Autodesk Inventor part; units mm, degrees
ref_plane "Work Plane2" through (0, 10, 0) normal (0, 1, 0) x (1, 0, 0)
ref_plane "YZ Plane" through (0, 0, 0) normal (1, 0, 0) x (0, 1, 0)
ref_plane "XZ Plane" through (0, 0, 0) normal (0, 1, 0) x (-1, 0, 0)
sketch "Sketch1" plane through (0, 0, 0) normal (0, 1, 0) x (-1, 0, 0)
  circle A0 centre (0, 0) radius 66
  circle A1 centre (0, 0) radius 61
  circle A2 centre (0, 0) radius 59
  dimension "Absolute_Diameter" = 132
  dimension "Diameter_No_Outer_Lip" = 122
  dimension "Inner_Cylinder_Diameter" = 118
extrude "Extrusion1" add sketch "Sketch1" along normal blind 4 contours A0
extrude "Extrusion2" add sketch "Sketch1" along normal blind 75 contours A1
sketch "Sketch2" plane through (0, 75, 0) normal (0, 1, 0) x (1, 0, 0)
  circle A0 centre (0, 0) radius 40.5
  circle A1 centre (0, 0) radius 61
  dimension "Lip_Diameter_Out" = 81
  dimension "Top_Outer_Lip_Diameter" = 122
extrude "Extrusion7" add sketch "Sketch2" against normal blind 8
ref_plane "Work Plane2" through (0, 10, 0) normal (0, 1, 0) x (1, 0, 0)
sketch "Sketch3" plane through (0, 10, 0) normal (0, 1, 0) x (1, 0, 0)
  circle A0 centre (0, 0) radius 127.5
  circle A1 centre (-127.5, 0) radius 2.5
  circle A2 centre (-103.1497, -74.9426) radius 2.5
  circle A3 centre (-39.3997, -121.2597) radius 2.5
  circle A4 centre (39.3997, -121.2597) radius 2.5
  circle A5 centre (103.1497, -74.9426) radius 2.5
  circle A6 centre (127.5, 0) radius 2.5
  circle A7 centre (103.1497, 74.9426) radius 2.5
  circle A8 centre (39.3997, 121.2597) radius 2.5
  circle A9 centre (-39.3997, 121.2597) radius 2.5
  circle A10 centre (-103.1497, 74.9426) radius 2.5
  dimension "d27" = 255
  dimension "d28" = 5
  dimension "d31" = 360
extrude "Extrusion8" [suppressed]
sketch "Sketch24" plane through (0, 75, 0) normal (0, 1, 0) x (1, 0, 0)
  circle A0 centre (0, 0) radius 51
  circle A1 centre (0, -51) radius 2.75
  circle A2 centre (44.1673, -25.5) radius 2.75
  circle A3 centre (44.1673, 25.5) radius 2.75
  circle A4 centre (0, 51) radius 2.75
  circle A5 centre (-44.1673, 25.5) radius 2.75
  circle A6 centre (-44.1673, -25.5) radius 2.75
  dimension "d230" = 102
  dimension "d231" = 5.5
  dimension "d234" = 360
extrude "Extrusion30" cut sketch "Sketch24" against normal blind 10 contours A3 A0 | A0 A3 | A2 A0 | A0 A2 | A4 A0 | A0 A4 | A1 A0 | A0 A1 | A5 A0 | A0 A5 | A6 A0 | A0 A6
properties part number "Cylinder Replacement- 11"
Check sheet for the modelled part. Datum: model origin and axes. Units: mm. A direction names the side the tool comes from. Round coordinates to 2 decimals unless told otherwise and drop trailing zeros. Write each loop counter-clockwise with the first axis right and the second up, starting at its lowest first coordinate (ties: lowest second). Pieces come first, ordered by that corner, then holes. Notation, with made-up numbers: (-37, 63.25) - (-19, 63.25) arc R15 ccw to (-19, 92.25) - close; hole circle Ø4 at (-10, 74.25). An arc over 180 degrees is marked (long way). Return JSON: item names as keys, results as strings.
Q1. Draft check along X on faces 4 (the flat face through (-40, 75, -13)), 5 (the cylindrical face through (-56.275, 33.031, -17.722)), 6 (the cylindrical face through (42.14, 71.06, -27.36)), 7 (the cylindrical face through (48.408, 39.003, 37.118)). Enter one of: released by +X, released by -X, zero draft, split by the parting line, or undercut.
Returned:
{"face 4": "zero draft", "face 5": "undercut", "face 6": "undercut", "face 7": "split by the parting line"}
Q2. Depth check by flat-ended pin: P1, Ø3.5, axis at x = 0, z = 51, coming from the +Y side; P2, Ø1.5, axis at y = 60.5, z = 29, coming from the -X side; P3, Ø12, axis at y = 47, z = 8.5, coming from the +X side; P4, Ø10, axis at x = 16.5, y = 48, coming from the -Z side. Enter the tip coordinate at first touch or a pass-through.
Returned:
{"P1": "passes through", "P2": "stops at x = -54.06", "P3": "stops at x = 60.95", "P4": "stops at z = -59.91"}
Q3. Cross-section at B-B (z = 0). Record the boundary of the cut face in (x, y).
Returned:
{"outline": "(-66, 0) - (-59, 0) - (-59, 67) - (-40.5, 67) - (-40.5, 75) - (-61, 75) - (-61, 4) - (-66, 4) - close; (40.5, 67) - (59, 67) - (59, 0) - (66, 0) - (66, 4) - (61, 4) - (61, 75) - (40.5, 75) - close"}
Q4. Access from +Z, -Z, +X, -X, +Y, -Y to the whole of each face (thin tool, end or side, straight path). Record for faces 1 (the flat face through (-58.4, 4, -19.2)), 2 (the cylindrical face through (-46.915, 71.056, -25.621)), 3 (the flat face through (-14, 67, 39)).
Returned:
{"face 1": "+Y", "face 2": "+Y, -Y", "face 3": "-Y"}
Q5. Cross-section at D-D (x = -33.5). Record the boundary of the cut face in (y, z), then the cut area to 3 significant figures.
Returned:
{"outline": "(0, -56.87) - (4, -56.87) - (4, -50.98) - (75, -50.98) - (75, -22.76) - (67, -22.76) - (67, -48.57) - (0, -48.57) - close; (0, 48.57) - (67, 48.57) - (67, 22.76) - (75, 22.76) - (75, 50.98) - (4, 50.98) - (4, 56.87) - (0, 56.87) - close", "area": "822 mm²"}
Q6. Scan lines: L1, parallel to Z at x = 0, y = 73; L2, parallel to X at y = 71, z = -25; L3, parallel to X at y = 60, z = 0.5. Record each from-to range of solid material in increasing order. Write a range as from..to.
Returned:
{"L1": "z = -61..-53.75, -48.25..-40.5, 40.5..48.25, 53.75..61", "L2": "x = -55.64..-46.87, -41.46..-31.86, 31.86..41.46, 46.87..55.64", "L3": "x = -61..-59, 59..61"}
Q7. Cross-section at A-A (x = 0). Record the boundary of the cut face in (y, z), then the cut area to 3 significant figures.
Returned:
{"outline": "(0, -66) - (4, -66) - (4, -61) - (75, -61) - (75, -53.75) - (67, -53.75) - (67, -59) - (0, -59) - close; (0, 59) - (67, 59) - (67, 53.75) - (75, 53.75) - (75, 61) - (4, 61) - (4, 66) - (0, 66) - close; (67, -48.25) - (75, -48.25) - (75, -40.5) - (67, -40.5) - close; (67, 40.5) - (75, 40.5) - (75, 48.25) - (67, 48.25) - close", "area": "548 mm²"}
Q8. Cross-section at C-C (y = 33). Record the boundary of the cut face in (x, z), then the cut area to 3 significant figures.
Returned:
{"outline": "circle Ø122 at (0, 0); hole circle Ø118 at (0, 0)", "area": "754 mm²"}
